The listing builds one solid part. Answer for the finished solid, in the listing's coordinates (mm). Round coordinates to 2 decimals unless told otherwise and drop trailing zeros. Write each loop counter-clockwise with the first axis right and the second up, starting at its lowest first coordinate (ties: lowest second). Pieces come first, ordered by that corner, then holes.
from build123d import *

# Parameters (mm, degrees)
SKETCH1_W                  = 92.5
SKETCH1_H                  = 92.5
BOSS_EXTRUDE1_DEPTH        = 1.5
F_3_1_3_1_DIAMETER_HOLE1_D = 3.1
SKETCH4_W                  = 1.5
SKETCH4_H                  = 69.5
SKETCH4_W_2                = 69.5
SKETCH4_H_2                = 1.5
CUT_EXTRUDE1_DEPTH         = 10


with BuildPart() as part:
    # Sketch1 → Boss-Extrude1 (new body)
    with BuildSketch(Plane.XY):
        Rectangle(SKETCH1_W, SKETCH1_H)
    extrude(amount=BOSS_EXTRUDE1_DEPTH)

    # Ø3.1 (3.1) Diameter Hole1 (through all)
    with Locations(Plane.XY.offset(1.5)):
        with Locations((-41.5, 41.5), (41.5, 41.5), (44.05, -37.33), (-41.5, -41.5)):
            Hole(F_3_1_3_1_DIAMETER_HOLE1_D / 2)

    # Sketch4 → Cut-Extrude1 (cut)
    with BuildSketch(Plane(origin=(0, 0, 0), x_dir=(-1, 0, 0), z_dir=(0, 0, -1))):
        with Locations((-45.5, 0)):
            Rectangle(SKETCH4_W, SKETCH4_H)
        with Locations((45.5, 0)):
            Rectangle(SKETCH4_W, SKETCH4_H)
        with Locations((0, 45.5)):
            Rectangle(SKETCH4_W_2, SKETCH4_H_2)
    extrude(amount=-CUT_EXTRUDE1_DEPTH, mode=Mode.SUBTRACT)


solid = part.part
1. Section B-B on z = 1 is taken. Determine the outline of the cut face in (x, y), plus the area to 3 significant figures.
Geometry says:
outline: (-46.25, -46.25) - (46.25, -46.25) - (46.25, -34.75) - (44.75, -34.75) - (44.75, 34.75) - (46.25, 34.75) - (46.25, 46.25) - (34.75, 46.25) - (34.75, 44.75) - (-34.75, 44.75) - (-34.75, 46.25) - (-46.25, 46.25) - (-46.25, 34.75) - (-44.75, 34.75) - (-44.75, -34.75) - (-46.25, -34.75) - close; hole circle Ø3.1 at (-41.5, -41.5); hole circle Ø3.1 at (-41.5, 41.5); hole circle Ø3.1 at (41.5, 41.5); hole circle Ø3.1 at (44.05, -37.33)
area: 8,210 mm2
2. For a pull along Y with two mould halves and no side action, classify faces 1 (the face through (-42.215, -42.875, 0.739)), 2 (the face through (-1, 1, 0)) as released by +Y, released by -Y, zero draft, split by the parting line, or undercut.
Geometry says:
face 1: undercut
face 2: zero draft
3. Section C-C on y = -37.33 is taken. Determine the outline of the cut face in (x, z).
Geometry says:
outline: (-46.25, 0) - (42.5, 0) - (42.5, 1.5) - (-46.25, 1.5) - close; (45.6, 0) - (46.25, 0) - (46.25, 1.5) - (45.6, 1.5) - close
4. Given pin 1 (0.8 mm diameter, centred on y = 9.5, z = 0.5, fed in from -X); pin 2 (5 mm diameter, centred on x = -41.5, y = -41.5, fed in from +Z), each flat-ended and moving along its own axis, determine where each tip first touches the part or whether it passes through.
Geometry says:
pin 1: stops at x = -44.75
pin 2: stops at z = 1.5
5. Section A-A on y = 41.5 is taken. Determine the outline of the cut face in (x, z).
Geometry says:
outline: (-46.25, 0) - (-43.05, 0) - (-43.05, 1.5) - (-46.25, 1.5) - close; (-39.95, 0) - (39.95, 0) - (39.95, 1.5) - (-39.95, 1.5) - close; (43.05, 0) - (46.25, 0) - (46.25, 1.5) - (43.05, 1.5) - close
6. Straight lines are drawn through the part: line 1 along Y through (x, z) = (-41.5, 0.85); line 2 along X through (y, z) = (17, 0.7); line 3 along Y through (x, z) = (13, 0.65). For each, find the intervals that lie inside material, in ascending order.
Geometry says:
line 1: y = -46.25 to -43.05, -39.95 to 39.95, 43.05 to 46.25
line 2: x = -44.75 to 44.75
line 3: y = -46.25 to 44.75
